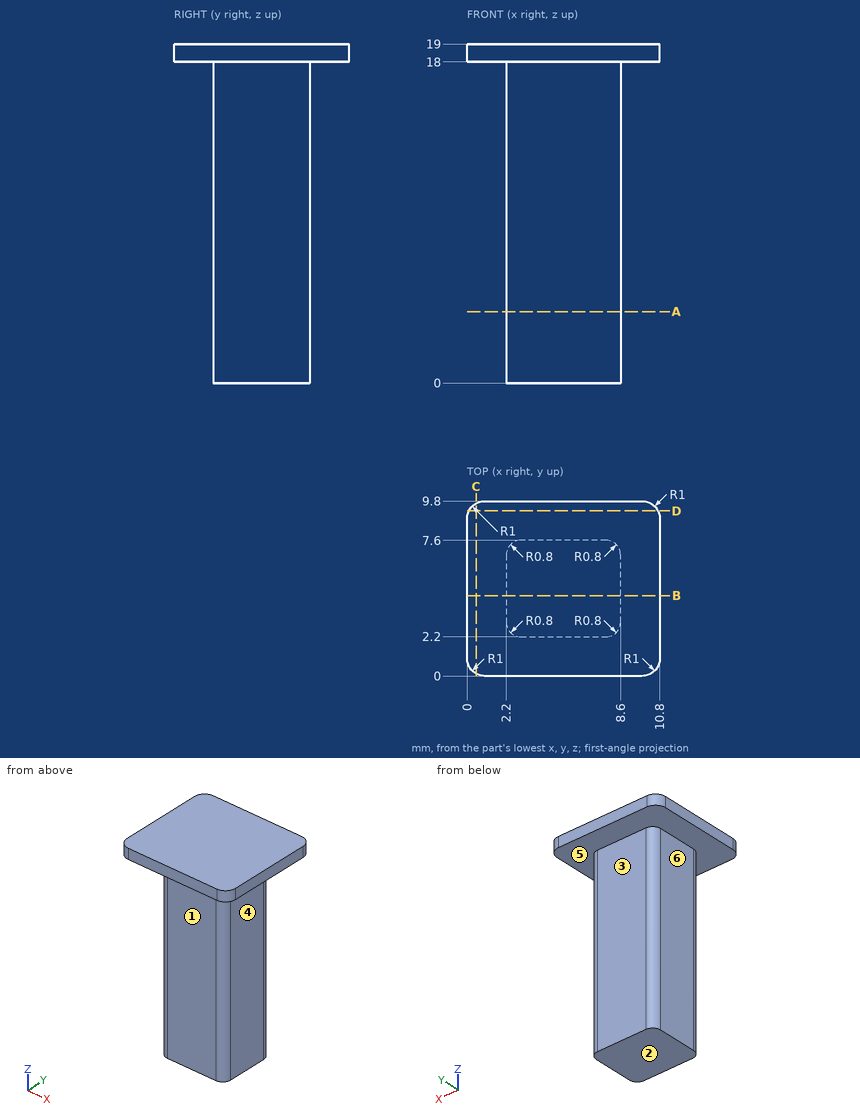
Part print with two shaded views. Sizes in mm from the minimum x, y, z corner. A direction names the side the tool comes from. Coordinates: 2 decimals unless noted, no trailing zeros. Order: outer loops, then holes, each group sorted by start corner. A loop starts at its lowest first (then second) coordinate and runs counter-clockwise, first axis right, second up. Notation, with made-up numbers: (20, 76) - (63, 76) arc R10 cw to (63, 92) - close; hole circle Ø11 at (-9.75, 64.5). An arc over 180 degrees is marked (long way). Answer in a Markdown table with one row per item.
1. Slice it at B-B, the plane y = 4.5. List the corners of the cut face in (x, z), then the cut area to 3 significant figures.
Answer:
| item | result |
|---|---|
| outline | (0, 18) - (2.2, 18) - (2.2, 0) - (8.6, 0) - (8.6, 18) - (10.8, 18) - (10.8, 19) - (0, 19) - close |
| area | 126 mm² |
2. Slice it at C-C, the plane x = 0.5. List the corners of the cut face in (y, z).
Answer:
| item | result |
|---|---|
| outline | (0.13, 18) - (9.67, 18) - (9.67, 19) - (0.13, 19) - close |
3. Flat gauge pins, fed straight in: P1, Ø3, axis at x = 9.5, z = 2.5, coming from the +Y side; P2, Ø5, axis at x = 9.5, z = 12.5, coming from the -Y side; P3, Ø1, axis at y = 7, z = 15.5, coming from the +X side. Where does each tip first touch, or does it go through?
Answer:
| item | result |
|---|---|
| P1 | y = 7.57 |
| P2 | y = 2.2 |
| P3 | x = 8.6 |
4. Pull direction X, two halves, no side cores. Call the marked faces 4, 5 and 6: +X half, -X half, draft (parallel to the pull), parting line (faces both ways), or undercut.
Answer:
| item | result |
|---|---|
| face 4 | +X half |
| face 5 | draft |
| face 6 | -X half |
5. Slice it at A-A, the plane z = 4. List the corners of the cut face in (x, y).
Answer:
| item | result |
|---|---|
| outline | (2.2, 3) arc R0.8 ccw to (3, 2.2) - (7.8, 2.2) arc R0.8 ccw to (8.6, 3) - (8.6, 6.8) arc R0.8 ccw to (7.8, 7.6) - (3, 7.6) arc R0.8 ccw to (2.2, 6.8) - close |
6. Slice it at D-D, the plane y = 9.25. List the corners of the cut face in (x, z).
Answer:
| item | result |
|---|---|
| outline | (0.11, 18) - (10.69, 18) - (10.69, 19) - (0.11, 19) - close |
7. Drill centre lines: L1, parallel to Y at x = 6, z = 11.5; L2, parallel to Z at x = 7.5, y = 9.5; L3, parallel to X at y = 6.5, z = 2.5. Where is each one in solid material? Low to high. Write a range as from..to.
Answer:
| item | result |
|---|---|
| L1 | 2.2..7.6 |
| L2 | 18..19 |
| L3 | 2.2..8.6 |
8. 3-axis set-ups, long thin cutter, end or side, ignore diameter. For the marked faces 1, 2 and 3: which of +Z, -Z, +X, -X, +Y, -Y reach the whole face in a straight line?
Answer:
| item | result |
|---|---|
| face 1 | -Z, +X, -X, -Y |
| face 2 | -Z, +X, -X, +Y, -Y |
| face 3 | -Z, +X, -X, +Y |
